Here's the drawing with two shaded views (mm, measured from the low corner). I have some questions. Round coordinates to 2 decimals unless told otherwise and drop trailing zeros. Order: outer loops, then holes, each group sorted by start corner. A loop starts at its lowest first (then second) coordinate and runs counter-clockwise, first axis right, second up.
Q1. If we section it at D-D (x = 50.5): Please give me the cut outline in (y, z), plus the area to 3 significant figures.
Q2. If we section it at A-A (x = 39.5): Please give me the cut outline in (y, z), plus the area to 3 significant figures.
Q3. Will these pins go through, and if not, where does the flat tip stop? P1, Ø1.5, axis at y = 71, z = 1, coming from the +X side; P2, Ø1.5, axis at x = 39, z = 1, coming from the -Y side; P3, Ø0.9, axis at x = 74, z = 1, coming from the +Y side.
Q4. If we section it at B-B (z = 1.35): Please give me the cut outline in (x, y), plus the area to 3 significant figures.
Q5. If we section it at C-C (y = 74): Please give me the cut outline in (x, z), plus the area to 3 significant figures.
Q6. If I drill on line 1 (Y direction, x = 51.5, z = 2.6); line 2 (X direction, y = 60.5, z = 2.1); line 3 (Y direction, x = 28, z = 2.1), over which ranges is the centre line in solid material (lowest first)?
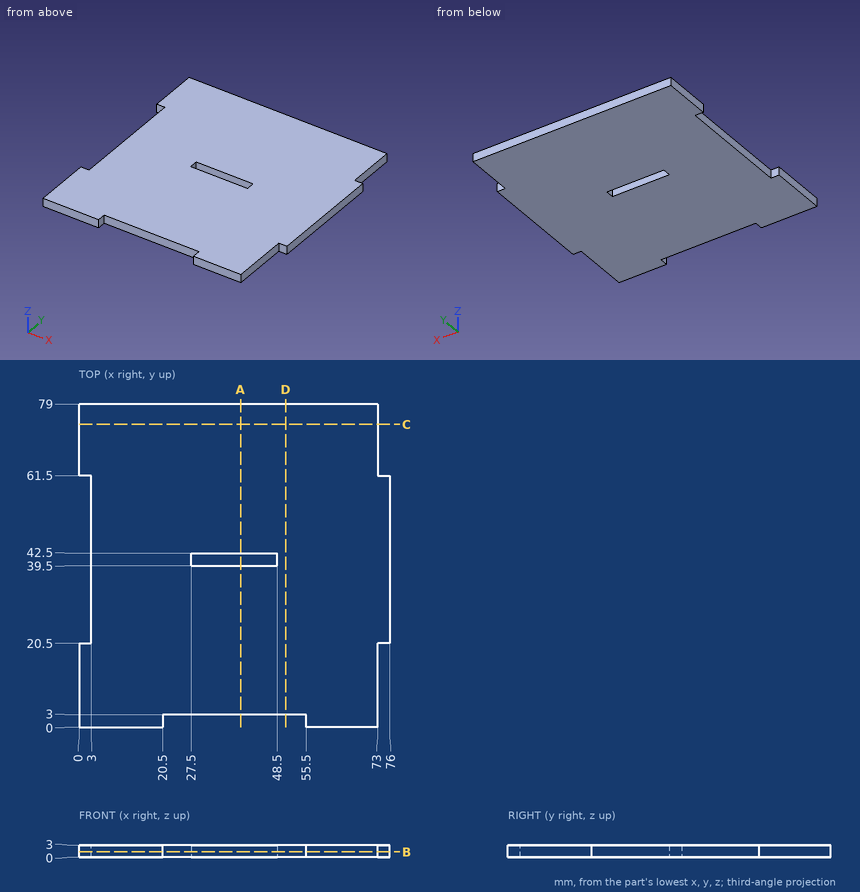
Solution:
1. outline: (3, 0) - (79, 0) - (79, 3) - (3, 3) - close
1. area: 228 mm2
2. outline: (3, 0) - (39.5, 0) - (39.5, 3) - (3, 3) - close; (42.5, 0) - (79, 0) - (79, 3) - (42.5, 3) - close
2. area: 219 mm2
3. P1: stops at x = 73
3. P2: stops at y = 3
3. P3: stops at y = 61.5
4. outline: (0, 0) - (20.5, 0) - (20.5, 3) - (55.5, 3) - (55.5, 0) - (73, 0) - (73, 20.5) - (76, 20.5) - (76, 61.5) - (73, 61.5) - (73, 79) - (0, 79) - (0, 61.5) - (3, 61.5) - (3, 20.5) - (0, 20.5) - close; hole (27.5, 39.5) - (48.5, 39.5) - (48.5, 42.5) - (27.5, 42.5) - close
4. area: 5,600 mm2
5. outline: (0, 0) - (73, 0) - (73, 3) - (0, 3) - close
5. area: 219 mm2
6. line 1: y = 3 to 79
6. line 2: x = 3 to 76
6. line 3: y = 3 to 39.5, 42.5 to 79
